from build123d import *

# Parameters (mm, degrees)
BOSS_EXTRUDE3_DEPTH     = 45
CUT_EXTRUDE1_DEPTH      = 201.870207973
CUT_EXTRUDE1_DEPTH_BACK = 201.870207973
BOSS_EXTRUDE10_DEPTH    = 45
CUT_EXTRUDE2_DEPTH      = 201.870207973
CUT_EXTRUDE3_DEPTH      = 189.545324927
SKETCH14_W              = 5
SKETCH14_H              = 30.172848437
CUT_EXTRUDE4_DEPTH      = 5
FILLET2_R               = 15
FILLET4_R               = 10
CUT_EXTRUDE5_DEPTH      = 4


with BuildPart() as part:
    # Sketch4 → Boss-Extrude3 (new body)
    with BuildSketch(Plane(origin=(0, 0, 0), x_dir=(1, 0, 0), z_dir=(0, 1, 0))):
        Polygon((0, 49.75), (-34.996508397, 87.75), (174.996508397, 87.75), (140, 49.75), (140, 0), (0, 0), align=None)
    extrude(amount=BOSS_EXTRUDE3_DEPTH)

    # Sketch5 → Cut-Extrude1 (cut, two sides: drawn at the far end of the back side and taken through both)
    with BuildSketch(Plane(origin=(140, 0, 0), x_dir=(0, 0, -1), z_dir=(1, 0, 0)).offset(-CUT_EXTRUDE1_DEPTH_BACK)):
        Polygon((0, 45), (3, 2), (49.75, 3), (87.75, 0), (87.75, 45), align=None)
    extrude(amount=CUT_EXTRUDE1_DEPTH + CUT_EXTRUDE1_DEPTH_BACK, mode=Mode.SUBTRACT)

    # Sketch12 → Boss-Extrude10 (add)
    with BuildSketch(Plane.XZ):
        Polygon((140, 0), (135, 0), (135, -51.701623266), (161.738177617, -80.734541004), (174.996508397, -87.75), (140, -49.75), align=None)
    boss_extrude10 = extrude(amount=-BOSS_EXTRUDE10_DEPTH)

    # Sketch6 → Cut-Extrude2 (cut, symmetric)
    with BuildSketch(Plane(origin=(140, 0, 0), x_dir=(0, 0, -1), z_dir=(1, 0, 0))):
        Polygon((49.75, 45), (0, 45), (31.854288426, 21.809847033), (49.75, 14.827151563), align=None)
    cut_extrude2 = extrude(amount=CUT_EXTRUDE2_DEPTH, both=True, mode=Mode.SUBTRACT)

    # Sketch13 → Cut-Extrude3 (cut, symmetric)
    with BuildSketch(Plane(origin=(50.959743513, 0, 46.931923468), x_dir=(0.6774391869389724, 0, -0.7355787843592718), z_dir=(0.7355787843592718, 0, 0.6774391869389724))):
        Polygon((131.436530693, 14.827151563), (183.096530693, 0), (183.096530693, 45), (131.436530693, 45), align=None)
    cut_extrude3 = extrude(amount=CUT_EXTRUDE3_DEPTH, both=True, mode=Mode.SUBTRACT)

    # Sketch14 → Cut-Extrude4 (cut)
    with BuildSketch(Plane(origin=(89.040256487, 0, -96.681923468), x_dir=(-0.7355787843592717, 0, -0.6774391869389725), z_dir=(0.6774391869389725, 0, -0.7355787843592717))):
        with Locations((-66.77843026, 29.913575782)):
            Rectangle(SKETCH14_W, SKETCH14_H)
    cut_extrude4 = extrude(amount=-CUT_EXTRUDE4_DEPTH, mode=Mode.SUBTRACT)

    # Mirror1: Boss-Extrude10, Cut-Extrude2, Cut-Extrude3, Cut-Extrude4 across plane
    add(boss_extrude10.mirror(Plane(origin=(70, 0, 0), x_dir=(0, 0, 1), z_dir=(1, 0, 0))))
    add(cut_extrude2.mirror(Plane(origin=(70, 0, 0), x_dir=(0, 0, 1), z_dir=(1, 0, 0))), mode=Mode.SUBTRACT)
    add(cut_extrude3.mirror(Plane(origin=(70, 0, 0), x_dir=(0, 0, 1), z_dir=(1, 0, 0))), mode=Mode.SUBTRACT)
    add(cut_extrude4.mirror(Plane(origin=(70, 0, 0), x_dir=(0, 0, 1), z_dir=(1, 0, 0))), mode=Mode.SUBTRACT)

    # Fillet2
    # the kernel refuses this fillet: 15 mm, written as the material it adds along each edge
    with BuildSketch(Plane(origin=(5, -35.409066281, -5.609934857), x_dir=(1, 0, 0), z_dir=(0, 0.9975751008362208, 0.06959826284903867))) as fillet2_piece_1_section:
        with BuildLine():
            CenterArc((FILLET2_R, FILLET2_R), FILLET2_R, 180, 90)
            Line((0, FILLET2_R), (0, 0))
            Line((0, 0), (FILLET2_R, 0))
        make_face()
    fillet2_piece_1 = extrude(amount=118.104524125, mode=Mode.PRIVATE)
    fillet2_piece_1 = split(fillet2_piece_1, bisect_by=Plane(origin=(8.441655444, 34.86103845, -13.92700626), z_dir=(0, -0.808453521145491, 0.5885600259510132)), keep=Keep.TOP, mode=Mode.PRIVATE)
    fillet2_piece_1 = split(fillet2_piece_1, bisect_by=Plane(origin=(8.441655444, 0, -4.786685936), z_dir=(0, 1, 0)), keep=Keep.TOP, mode=Mode.PRIVATE)
    add(fillet2_piece_1)
    with BuildSketch(Plane(origin=(135, -35.409066281, -5.609934857), x_dir=(-1, 0, 0), z_dir=(0, 0.9975751008362208, 0.06959826284903867))) as fillet2_piece_2_section:
        with BuildLine():
            CenterArc((FILLET2_R, -FILLET2_R), FILLET2_R, 90, 90)
            Line((0, -FILLET2_R), (0, 0))
            Line((0, 0), (FILLET2_R, 0))
        make_face()
    fillet2_piece_2 = extrude(amount=118.104524125, mode=Mode.PRIVATE)
    fillet2_piece_2 = split(fillet2_piece_2, bisect_by=Plane(origin=(131.558344556, 34.86103845, -13.92700626), z_dir=(0, -0.808453521145491, 0.5885600259510132)), keep=Keep.TOP, mode=Mode.PRIVATE)
    fillet2_piece_2 = split(fillet2_piece_2, bisect_by=Plane(origin=(131.558344556, 0, -4.786685936), z_dir=(0, 1, 0)), keep=Keep.TOP, mode=Mode.PRIVATE)
    add(fillet2_piece_2)
    with BuildSketch(Plane(origin=(5, 2, -3), x_dir=(0, 0.9975751008362208, 0.06959826284903871), z_dir=(1, 0, 0))) as fillet2_piece_3_section:
        with BuildLine():
            CenterArc((FILLET2_R * 0.952861026227, -FILLET2_R), FILLET2_R, 90, 87.234478204)
            Line((-FILLET2_R * 0.0459743260206, -FILLET2_R * 0.951751278775), (0, 0))
            Line((0, 0), (FILLET2_R * 0.952861026227, 0))
        make_face()
    fillet2_piece_3 = extrude(amount=165.732288484, mode=Mode.PRIVATE)
    fillet2_piece_3 = split(fillet2_piece_3, bisect_by=Plane(origin=(140, 5.230522006, -5.949029167), z_dir=(-1, 0, 0)), keep=Keep.TOP, mode=Mode.PRIVATE)
    add(fillet2_piece_3)
    # the kernel refuses this fillet: 15 mm, written as the material it takes off along each edge
    with BuildSketch(Plane(origin=(-21.738177617, -5.880130796, -80.734541004), x_dir=(-0.8838887186878241, 0, -0.4676972663768696), z_dir=(0, 1, 0))) as fillet2_2_piece_1_section:
        with BuildLine():
            CenterArc((FILLET2_R * 0.171572875254, FILLET2_R), FILLET2_R, 250.528779366, 19.471220634)
            Line((-FILLET2_R * 0.16176045808, FILLET2_R * 0.0571909584179), (0, 0))
            Line((0, 0), (FILLET2_R * 0.171572875254, 0))
        make_face()
    fillet2_2_piece_1 = extrude(amount=16.37310681, mode=Mode.PRIVATE)
    fillet2_2_piece_1 = split(fillet2_2_piece_1, bisect_by=Plane(origin=(-21.810642067, 0.577757784, -80.431734736), z_dir=(0, 0.9968981486534686, -0.07870248542001068)), keep=Keep.TOP, mode=Mode.PRIVATE)
    add(fillet2_2_piece_1, mode=Mode.SUBTRACT)
    with BuildSketch(Plane(origin=(5, -11.791250012, -51.701623266), x_dir=(-0.6774391869389725, 0, -0.7355787843592716), z_dir=(0, 1, 0))) as fillet2_2_piece_2_section:
        with BuildLine():
            CenterArc((FILLET2_R * 0.390324653104, FILLET2_R), FILLET2_R, 227.356145275, 42.643854725)
            Line((-FILLET2_R * 0.287114533835, FILLET2_R * 0.264421215641), (0, 0))
            Line((0, 0), (FILLET2_R * 0.390324653104, 0))
        make_face()
    fillet2_2_piece_2 = extrude(amount=41.255576067, mode=Mode.PRIVATE)
    fillet2_2_piece_2 = split(fillet2_2_piece_2, bisect_by=Plane(origin=(4.876560205, 2.973184578, -48.496379006), z_dir=(0, 0.9997713044194101, 0.021385482447473975)), keep=Keep.TOP, mode=Mode.PRIVATE)
    add(fillet2_2_piece_2, mode=Mode.SUBTRACT)
    with BuildSketch(Plane(origin=(5, -11.791250012, -51.701623266), x_dir=(-0.6774391869389725, 0, -0.7355787843592716), z_dir=(0, 1, 0))) as fillet2_2_piece_3_section:
        with BuildLine():
            CenterArc((FILLET2_R * 0.390324653104, FILLET2_R), FILLET2_R, 227.356145275, 42.643854725)
            Line((-FILLET2_R * 0.287114533835, FILLET2_R * 0.264421215641), (0, 0))
            Line((0, 0), (FILLET2_R * 0.390324653104, 0))
        make_face()
    fillet2_2_piece_3 = extrude(amount=41.255576067, mode=Mode.PRIVATE)
    fillet2_2_piece_3 = split(fillet2_2_piece_3, bisect_by=Plane(origin=(3.697267627, 2.777037551, -52.574191023), z_dir=(0, 0.9968981486534686, -0.07870248542001068)), keep=Keep.TOP, mode=Mode.PRIVATE)
    add(fillet2_2_piece_3, mode=Mode.SUBTRACT)
    with BuildSketch(Plane(origin=(161.738177617, -5.880130796, -80.734541004), x_dir=(-0.6774391869389714, 0, 0.7355787843592727), z_dir=(0, 1, 0))) as fillet2_2_piece_4_section:
        with BuildLine():
            CenterArc((FILLET2_R * 0.171572875254, FILLET2_R), FILLET2_R, 250.528779366, 19.471220634)
            Line((-FILLET2_R * 0.16176045808, FILLET2_R * 0.0571909584179), (0, 0))
            Line((0, 0), (FILLET2_R * 0.171572875254, 0))
        make_face()
    fillet2_2_piece_4 = extrude(amount=16.37310681, mode=Mode.PRIVATE)
    fillet2_2_piece_4 = split(fillet2_2_piece_4, bisect_by=Plane(origin=(161.810642067, 0.577757784, -80.431734736), z_dir=(0, 0.9968981486534686, -0.07870248542001068)), keep=Keep.TOP, mode=Mode.PRIVATE)
    add(fillet2_2_piece_4, mode=Mode.SUBTRACT)
    with BuildSketch(Plane(origin=(135, -11.791250012, -51.701623266), x_dir=(0.6774391869389733, 0, -0.7355787843592709), z_dir=(0, 1, 0))) as fillet2_2_piece_5_section:
        with BuildLine():
            CenterArc((FILLET2_R * 0.390324653104, -FILLET2_R), FILLET2_R, 90, 42.643854725)
            Line((-FILLET2_R * 0.287114533835, -FILLET2_R * 0.264421215641), (0, 0))
            Line((0, 0), (FILLET2_R * 0.390324653104, 0))
        make_face()
    fillet2_2_piece_5 = extrude(amount=41.255576067, mode=Mode.PRIVATE)
    fillet2_2_piece_5 = split(fillet2_2_piece_5, bisect_by=Plane(origin=(135.123439795, 2.973184578, -48.496379006), z_dir=(0, 0.9997713044194101, 0.021385482447473975)), keep=Keep.TOP, mode=Mode.PRIVATE)
    add(fillet2_2_piece_5, mode=Mode.SUBTRACT)
    with BuildSketch(Plane(origin=(135, -11.791250012, -51.701623266), x_dir=(0.6774391869389733, 0, -0.7355787843592709), z_dir=(0, 1, 0))) as fillet2_2_piece_6_section:
        with BuildLine():
            CenterArc((FILLET2_R * 0.390324653104, -FILLET2_R), FILLET2_R, 90, 42.643854725)
            Line((-FILLET2_R * 0.287114533835, -FILLET2_R * 0.264421215641), (0, 0))
            Line((0, 0), (FILLET2_R * 0.390324653104, 0))
        make_face()
    fillet2_2_piece_6 = extrude(amount=41.255576067, mode=Mode.PRIVATE)
    fillet2_2_piece_6 = split(fillet2_2_piece_6, bisect_by=Plane(origin=(136.302732373, 2.777037551, -52.574191023), z_dir=(0, 0.9968981486534686, -0.07870248542001068)), keep=Keep.TOP, mode=Mode.PRIVATE)
    add(fillet2_2_piece_6, mode=Mode.SUBTRACT)

    # Fillet4
    fillet4_edges = [part.edges().sort_by_distance(p)[0] for p in [
        (70, 3, -49.75),
    ]]
    fillet(fillet4_edges, radius=FILLET4_R)

    # Sketch16 → Cut-Extrude5 (cut)
    with BuildSketch(Plane(origin=(140, 0, 0), x_dir=(0, 0, -1), z_dir=(1, 0, 0))):
        Polygon((0, 30.42), (0, 18), (13, 18), (20, 24.21), (13, 30.42), align=None)
    cut_extrude5 = extrude(amount=-CUT_EXTRUDE5_DEPTH, mode=Mode.SUBTRACT)

    # Mirror2: Cut-Extrude5 across plane
    add(cut_extrude5.mirror(Plane(origin=(70, 0, 0), x_dir=(0, 0, 1), z_dir=(1, 0, 0))), mode=Mode.SUBTRACT)


solid = part.part
Build history of the part. All positions in model axes, mm. A direction names the side the tool comes from. Round coordinates to 2 decimals unless told otherwise and drop trailing zeros. Loops run counter-clockwise (first coordinate to the right, second up) from the corner with the lowest first, then second, coordinate; pieces in that order, holes last. Notation, with made-up numbers: (5.25, 65) -> (9.25, 65) arc R24 ccw to (9.25, 86) -> close; hole circle Ø1 at (33, 73). An arc over 180 degrees is marked (long way). One line per item, written item: value. Start each with the question number.
Q1. Two-plate mould, pull along X, no slides. Class faces 4 (the face through (71, 0, -44)), 5 (the face through (4, 24, -8)), 6 (the face through (137, 14.827, -50)), 7 (the face through (149.966, 4.015, -60.572)): released by +X, released by -X, zero draft, split by the parting line, or undercut.
Q2. Drop flat-ended pins along their axis: pin 1 Ø2.5 at (x, z) = (3.5, -51) entering from +Y; pin 2 Ø9 at (y, z) = (15.5, -27.5) entering from +X; pin 3 Ø9 at (y, z) = (17.5, -35.5) entering from -X. Give the stop position or say it passes through.
Q3. Probe line 1 along X through (y, z) = (9, -47.5); line 2 along X through (y, z) = (20.5, -30.5); line 3 along Y through (x, z) = (34, -14.5). List the from-to ranges inside material, lowest first.
Q4. Cut at B-B on z = -39. List the corners of the cut face in (x, y).
Q5. 3-axis set-ups, long thin cutter, end or side, ignore diameter. For faces 1 (the face through (138, 30.42, -7)), 2 (the face through (4, 9.33, -51.23)), 3 (the face through (2, 30.42, -7)): which of +Z, -Z, +X, -X, +Y, -Y reach the whole face in a straight line?
Q6. Cut at C-C on x = 132.5. List the corners of the cut face in (y, z).
Q7. Cut at A-A on x = 39.5. List the corners of the cut face in (y, z).
Computed:
1. face 4: zero draft
1. face 5: released by -X
1. face 6: undercut
1. face 7: released by +X
2. pin 1: y = 14.83
2. pin 2: x = 140
2. pin 3: x = 0
3. line 1: 0 to 4.91, 135.09 to 140
3. line 2: 0 to 5, 135 to 140
3. line 3: 0 to 2.51
4. outline: (0, 0) -> (140, 0) -> (140, 19.02) -> (135, 19.02) -> (135, 2.77) -> (5, 2.77) -> (5, 19.02) -> (0, 19.02) -> close
5. face 1: +Z, +X
5. face 2: -Z, +Y
5. face 3: +Z, -X
6. outline: (0, -87.75) -> (2.96, -50.25) arc R10 ccw to (2.99, -49.25) -> (2.31, -17.29) arc R15 cw to (4.26, -9.57) -> (39.84, -7.08) -> (45, 0) -> (0, 0) -> close
7. outline: (0, -87.75) -> (2.96, -50.25) arc R10 ccw to (2.99, -49.25) -> (2.31, -17.29) arc R15 cw to (16.26, -2.01) -> (45, 0) -> (0, 0) -> close
